Model file for the job. Use its own axes, mm. A direction names the side the tool comes from. Give positions to 0.01 mm unless a question says otherwise; leave off trailing zeros. Write each loop counter-clockwise with the first axis right and the second up, starting at its lowest first coordinate (ties: lowest second). Pieces come first, ordered by that corner, then holes. Notation, with made-up numbers: (66.25, 8) - (92.25, 8) arc R18 cw to (92.25, 38) - close; hole circle Ø4 at (76.5, 43.25). An arc over 180 degrees is marked (long way). Use a Markdown table: item, result. Add a question column.
```python
from build123d import *

# Parameters (mm, degrees)
F0_R     = 4
F0_R_2   = 3
F1_DEPTH = 38
F2_R     = 4.25
F2_R_2   = 4
F2_R_3   = 3
F3_DEPTH = 0.5
F4_W     = 6.49
F4_H     = 2.75
F5_DEPTH = 12.5
F6_R     = 4
F6_R_2   = 3
F7_DEPTH = 2.5
F9_DEPTH = 6


with BuildPart() as f1:
    # F0 (on Front) → F1 (new body)
    with BuildSketch(Plane.XZ):
        Circle(F0_R)
        Circle(F0_R_2, mode=Mode.SUBTRACT)
    extrude(amount=-F1_DEPTH)

    # F2 (on face) → F3 (join)
    with BuildSketch(Plane.XZ):
        Circle(F2_R)
        Circle(F2_R_2, mode=Mode.SUBTRACT)
        Circle(F2_R_2)
        Circle(F2_R_3, mode=Mode.SUBTRACT)
    extrude(amount=-F3_DEPTH)

    # F4 (on Right) → F5 (cut, symmetric)
    with BuildSketch(Plane.YZ):
        with Locations((17.995, -2.625)):
            Rectangle(F4_W, F4_H)
    extrude(amount=F5_DEPTH, both=True, mode=Mode.SUBTRACT)

    # F6 (on face) → F7 (join)
    with BuildSketch(Plane(origin=(0, 38, 0), x_dir=(-1, 0, 0), z_dir=(0, 1, 0))):
        Circle(F6_R)
        Circle(F6_R_2, mode=Mode.SUBTRACT)
        Circle(F6_R_2)
    extrude(amount=-F7_DEPTH)

    # F8 (on face) → F9 (join)
    with BuildSketch(Plane(origin=(0, 38, 0), x_dir=(-1, 0, 0), z_dir=(0, 1, 0))):
        with BuildLine():
            Line((-1.1180339887, -1), (1.1180339887, -1))
            ThreePointArc((1.1180339887, -1), (0, 1.5), (-1.1180339887, -1))
        make_face()
    extrude(amount=F9_DEPTH)


solid = f1.part
```
(1) Two-plate mould, pull along X, no slides. Class faces 6 (the cylindrical face through (0, 18, 3)), 7 (the cylindrical face through (2.285, 0.246, 3.584)), 8 (the flat face through (0, 35.5, 0)), 9 (the flat face through (-3, 18, -1.25)): +X half, -X half, draft (parallel to the pull), parting line (faces both ways), or undercut.
(2) Flat gauge pins, fed straight in: pin 1 (4 mm diameter, centred on x = -1.5, y = 8.5, fed in from -Z); pin 2 (5 mm diameter, centred on x = -1.5, z = 1.5, fed in from -Y); pin 3 (2.5 mm diameter, centred on x = 0, y = 39.5, fed in from -Z); pin 4 (1.2 mm diameter, centred on x = -3, y = 19, fed in from -Z). Where does each tip first touch, or does it go through?
(3) Band-saw the part on D-D (y = 18). Write the cut outline in (x, z), then the cut area to 3 significant figures.
(4) Which spindle directions (+Z, -Z, +X, -X, +Y, -Y) get a long thin tool onto all of the face, cutting with end or side? Do faces 1 (the cylindrical face through (0, 41, 1.5)), 2 (the flat face through (1, 0, 3)), 3 (the flat face through (0, 44, 0)), 4 (the flat face through (3, 18, -1.25)), 5 (the flat face through (0, 41, -1)). Say none if no direction does.
(5) Band-saw the part on B-B (z = 0). Write the cut outline in (x, y).
(6) Band-saw the part on A-A (x = 0). Write the cut outline in (y, z).
(7) Band-saw the part on C-C (y = 7). Write the cut outline in (x, z), then the cut area to 3 significant figures.
(8) Probe probe 1 along Y at (x, z) = (2.75, -1.5); probe 2 along Z at (x, y) = (0, 24); probe 3 along Z at (x, y) = (0, 15). List the from-to ranges inside material, lowest first. Write a range as [from, to].
Model answer:
| question | item | result |
|---|---|---|
| 1 | face 6 | undercut |
| 1 | face 7 | parting line |
| 1 | face 8 | undercut |
| 1 | face 9 | draft |
| 2 | pin 1 | stops at z = -4 |
| 2 | pin 2 | stops at y = 0 |
| 2 | pin 3 | stops at z = -1 |
| 2 | pin 4 | stops at z = -1.25 |
| 3 | outline | (-3.8, -1.25) - (-2.73, -1.25) arc R3 cw (long way) to (2.73, -1.25) - (3.8, -1.25) arc R4 ccw (long way) to start |
| 3 | area | 13.6 mm^2 |
| 4 | face 1 | +Y |
| 4 | face 2 | +Z, -Z, +X, -X, -Y |
| 4 | face 3 | +Z, -Z, +X, -X, +Y |
| 4 | face 4 | -Z, +X, -X |
| 4 | face 5 | -Z, +X, -X, +Y |
| 5 | outline | (-4.25, 0) - (-3, 0) - (-3, 35.5) - (3, 35.5) - (3, 0) - (4.25, 0) - (4.25, 0.5) - (4, 0.5) - (4, 38) - (1.5, 38) - (1.5, 44) - (-1.5, 44) - (-1.5, 38) - (-4, 38) - (-4, 0.5) - (-4.25, 0.5) - close |
| 6 | outline | (0, -4.25) - (0.5, -4.25) - (0.5, -4) - (14.75, -4) - (14.75, -3) - (0, -3) - close; (0, 3) - (35.5, 3) - (35.5, -3) - (21.24, -3) - (21.24, -4) - (38, -4) - (38, -1) - (44, -1) - (44, 1.5) - (38, 1.5) - (38, 4) - (0.5, 4) - (0.5, 4.25) - (0, 4.25) - close |
| 7 | outline | circle Ø8 at (0, 0); hole circle Ø6 at (0, 0) |
| 7 | area | 22.0 mm^2 |
| 8 | probe 1 | y = [0, 14.75], [21.24, 38] |
| 8 | probe 2 | z = [-4, -3], [3, 4] |
| 8 | probe 3 | z = [3, 4] |
